Input: part model. Units: mm. Frame: model coordinates. A direction names the side the tool comes from. Coordinates: 2 decimals unless noted, no trailing zeros. Order: outer loops, then holes, each group sorted by start corner. A loop starts at its lowest first (then second) coordinate and runs counter-clockwise, first axis right, second up. Notation, with made-up numbers: M 29,65 L 80,65 A10 ccw 80,71 Z; hole C -23,-34.75 d5. An arc over 180 degrees is marked long. One line per item, written item: value.
Autodesk Inventor part; units mm, degrees
ref_plane "A4_XY" through (170, 0, 0) normal (0, 1, 0) x (1, 0, 0)
ref_plane "A4_YZ" through (170, 0, 0) normal (1, 0, 0) x (0, 0, -1)
ref_plane "A4_ZX" through (170, 0, 0) normal (0, 0, -1) x (0, 1, 0)
sketch "Sketch_1" plane through (0, 0, 0) normal (0, 0, 1) x (1, 0, 0)
  line L0 (67, 0) -> (-48, 0)
  line L1 (-48, 0) -> (-48, 4.233)
  line L2 (-48, 4.233) -> (-47.233, 5)
  line L3 (-47.233, 5) -> (-28.767, 5)
  line L4 (-28.767, 5) -> (-28, 4.233)
  line L5 (-28, 4.233) -> (-28, 4.2)
  line L6 (-28, 4.2) -> (-26, 4.2)
  line L7 (-26, 4.2) -> (-26, 5)
  line L8 (-26, 5) -> (-24.2679, 6)
  line L9 (-24.2679, 6) -> (57, 6)
  line L10 (57, 6) -> (57, 16)
  line L11 (57, 16) -> (67, 16)
  line L12 (67, 16) -> (67, 0)
  line L13 (67, 0) -> (-48, 0)
revolve "Revolution1" add sketch "Sketch_1" angle 360 about axis through (67, 0, 0) along (1, 0, 0)
thread "Thread1"
sketch "Sketch_4" plane through (-26, 0, 0) normal (1, 0, 0) x (0, 0, -1)
  line L0 (-13, -10) -> (13, -10)
  line L1 (13, -10) -> (13, 10)
  line L2 (13, 10) -> (-13, 10)
  line L3 (-13, 10) -> (-13, -10)
  line L4 (-8, 5) -> (-8, -5)
  line L5 (-8, -5) -> (8, -5)
  line L6 (8, -5) -> (8, 5)
  line L7 (8, 5) -> (-8, 5)
extrude "Extrusion1" cut sketch "Sketch_4" along normal blind 6
ref_plane "A4_XY" through (170, 0, 0) normal (0, 1, 0) x (1, 0, 0)
ref_plane "A4_YZ" through (170, 0, 0) normal (1, 0, 0) x (0, 0, -1)
ref_plane "A4_ZX" through (170, 0, 0) normal (0, 0, -1) x (0, 1, 0)
ref_plane "ROD_BODY_XY" through (0, 0, 0) normal (1, 0, 0) x (0, 0, -1)
ref_plane "ROD_BODY_YZ" through (0, 0, 0) normal (0, 0, -1) x (0, 1, 0)
ref_plane "ROD_BODY_ZX" through (0, 0, 0) normal (0, 1, 0) x (1, 0, 0)
ref_plane "ROD_NUT_XY" through (-48, 0, 0) normal (-1, 0, 0) x (0, 0, -1)
ref_plane "ROD_NUT_YZ" through (-48, 0, 0) normal (0, 0, -1) x (0, -1, 0)
ref_plane "ROD_NUT_ZX" through (-48, 0, 0) normal (0, -1, 0) x (-1, 0, 0)
properties part number "CP96S32-25_ROD"
(1) Ray query, line 1 (X direction, y = -7, z = -8); line 2 (Y direction, x = 40.5, z = 5); line 3 (Y direction, x = 30, z = -0.5). Return the intervals inside material, ascending. Write a range as from..to.
Data:
line 1: x = 57..67
line 2: y = -3.32..3.32
line 3: y = -5.98..5.98
(2) Cut plane B-B on x = -33. Output: boundary loops of the cut face in (y, z), plus the area to 3 significant figures.
Data:
outline: C 0,0 d10
area: 78.5 mm2
(3) Access query for faces 5 (the flat face through (-23, -5, 0)), 6 (the cylindrical face through (16.93, -0.78, 5.95)), 7 (the conical face through (-25.7, 0.11, 5.17)), 8 (the flat face through (-23, 5, 0)). Directions: +Z, -Z, +X, -X, +Y, -Y. A direction counts if a zero-diameter tool reaches every point of the face in a straight line with its end or side. Return the directions, or none.
Data:
face 5: +Z, -Z, -X, -Y
face 6: -X
face 7: +Z, -X
face 8: +Z, -Z, -X, +Y
(4) Cut plane D-D on x = 44.5. Output: boundary loops of the cut face in (y, z).
Data:
outline: C 0,0 d12
(5) Cut plane C-C on z = 10. Output: boundary loops of the cut face in (x, y).
Data:
outline: M 57,-12.49 L 67,-12.49 L 67,12.49 L 57,12.49 Z
(6) First-contact query: pin 1 (1 mm diameter, centred on y = 7.5, z = -5, fed in from -X); pin 2 (2 mm diameter, centred on x = 54.5, z = -12, fed in from +Y); pin 3 (0.5 mm diameter, centred on y = -5.5, z = -1, fed in from -X); pin 4 (4 mm diameter, centred on x = -2, y = 3, fed in from +Z). Flat tips, straight axial feed; report the tip coordinate or a pass-through.
Data:
pin 1: stops at x = 57
pin 2: passes through
pin 3: stops at x = -20
pin 4: stops at z = 5.92
(7) Draft query along X for faces 1 (the cylindrical face through (-37.87, -1.08, -4.88)), 2 (the conical face through (-25.7, -0.11, -5.17)), 3 (the flat face through (67, 0, 0)), 4 (the cylindrical face through (-26.986, 4.006, 1.262)). Return one class per face: released by +X, released by -X, zero draft, split by the parting line, or undercut.
Data:
face 1: zero draft
face 2: released by -X
face 3: released by +X
face 4: undercut
